```python
from build123d import *

# Parameters (mm, degrees)
F1_DEPTH    = 71.5
F0_R        = 0.8
F2_DEPTH    = 3
F3_T1_DEPTH = 18.8384580048
F3_T3_DEPTH = 18.8384580048
F3_T6_ANGLE = 198.9853445977
F3_T8_ANGLE = 161.0146554023
F6_W        = 6.8
F6_H        = 6.6
F7_DEPTH    = 10
F9_DEPTH    = 57.4


# Not quite as in the source:
# - a fillet or chamfer that OpenCascade refuses, or shapes differently, is made with other operations: its cross-section is extruded or revolved along the edge and cut away or added


with BuildPart() as f1:
    # F0 (on Top) → F1 (new body)
    with BuildSketch(Plane.XY):
        with BuildLine():
            ThreePointArc((10.5534817095, 15.4336250836), (0, 24.3689653978), (-10.5534817095, 15.4336250836))
            Line((-10.5534817095, 15.4336250836), (-13.6603478203, -3.1468722986))
            ThreePointArc((-13.6603478203, -3.1468722986), (0, -19.2810346022), (13.6603478203, -3.1468722986))
            Line((13.6603478203, -3.1468722986), (10.5534817095, 15.4336250836))
        make_face()
        with BuildLine():
            ThreePointArc((-12.1808877675, -3.3942544975), (-10.7458713669, 0.6557337165), (-8.0101498113, 3.9689653978))
            ThreePointArc((-8.0101498113, 3.9689653978), (-7.3298242511, 6.556361809), (-8.0101498113, 9.1437582202))
            ThreePointArc((-8.0101498113, 9.1437582202), (-9.0606365073, 12.0737017575), (-9.0740216568, 15.1862428847))
            ThreePointArc((-9.0740216568, 15.1862428847), (0, 22.8689653978), (9.0740216568, 15.1862428847))
            ThreePointArc((9.0740216568, 15.1862428847), (9.0606535532, 12.0737985759), (8.0102465186, 9.1439294077))
            ThreePointArc((8.0102465186, 9.1439294077), (8.0101981654, 9.1438438137), (8.0101498113, 9.1437582202))
            ThreePointArc((8.0101498113, 9.1437582202), (7.3298242511, 6.556361809), (8.0101498113, 3.9689653978))
            ThreePointArc((8.0101498113, 3.9689653978), (10.7458713669, 0.6557337165), (12.1808877675, -3.3942544975))
            ThreePointArc((12.1808877675, -3.3942544975), (0, -17.7810346022), (-12.1808877675, -3.3942544975))
        make_face(mode=Mode.SUBTRACT)
    extrude(amount=F1_DEPTH)

    # F0 (on Top) → F2 (join)
    with BuildSketch(Plane.XY):
        with BuildLine():
            ThreePointArc((10.5534817095, 15.4336250836), (0, 24.3689653978), (-10.5534817095, 15.4336250836))
            Line((-10.5534817095, 15.4336250836), (-13.6603478203, -3.1468722986))
            ThreePointArc((-13.6603478203, -3.1468722986), (0, -19.2810346022), (13.6603478203, -3.1468722986))
            Line((13.6603478203, -3.1468722986), (10.5534817095, 15.4336250836))
        make_face()
        with BuildLine():
            ThreePointArc((-12.1808877675, -3.3942544975), (-10.7458713669, 0.6557337165), (-8.0101498113, 3.9689653978))
            ThreePointArc((-8.0101498113, 3.9689653978), (-7.3298242511, 6.556361809), (-8.0101498113, 9.1437582202))
            ThreePointArc((-8.0101498113, 9.1437582202), (-9.0606365073, 12.0737017575), (-9.0740216568, 15.1862428847))
            ThreePointArc((-9.0740216568, 15.1862428847), (0, 22.8689653978), (9.0740216568, 15.1862428847))
            ThreePointArc((9.0740216568, 15.1862428847), (9.0606535532, 12.0737985759), (8.0102465186, 9.1439294077))
            ThreePointArc((8.0102465186, 9.1439294077), (8.0101981654, 9.1438438137), (8.0101498113, 9.1437582202))
            ThreePointArc((8.0101498113, 9.1437582202), (7.3298242511, 6.556361809), (8.0101498113, 3.9689653978))
            ThreePointArc((8.0101498113, 3.9689653978), (10.7458713669, 0.6557337165), (12.1808877675, -3.3942544975))
            ThreePointArc((12.1808877675, -3.3942544975), (0, -17.7810346022), (-12.1808877675, -3.3942544975))
        make_face(mode=Mode.SUBTRACT)
        with BuildLine():
            ThreePointArc((-9.0740216568, 15.1862428847), (-9.0606365073, 12.0737017575), (-8.0101498113, 9.1437582202))
            ThreePointArc((-8.0101498113, 9.1437582202), (0, 4.4689653978), (8.0101498113, 9.1437582202))
            ThreePointArc((8.0101498113, 9.1437582202), (8.0101981654, 9.1438438137), (8.0102465186, 9.1439294077))
            ThreePointArc((8.0102465186, 9.1439294077), (9.0606535532, 12.0737985759), (9.0740216568, 15.1862428847))
            ThreePointArc((9.0740216568, 15.1862428847), (0, 22.8689653978), (-9.0740216568, 15.1862428847))
        make_face()
        with BuildLine():
            ThreePointArc((-8.0101498113, 9.1437582202), (-7.3298242511, 6.556361809), (-8.0101498113, 3.9689653978))
            Line((-8.0101498113, 3.9689653978), (8.0101498113, 3.9689653978))
            ThreePointArc((8.0101498113, 3.9689653978), (7.3298242511, 6.556361809), (8.0101498113, 9.1437582202))
            ThreePointArc((8.0101498113, 9.1437582202), (0, 4.4689653978), (-8.0101498113, 9.1437582202))
        make_face()
        with BuildLine():
            Line((8.0101498113, 3.9689653978), (-8.0101498113, 3.9689653978))
            ThreePointArc((-8.0101498113, 3.9689653978), (-10.7458713669, 0.6557337165), (-12.1808877675, -3.3942544975))
            ThreePointArc((-12.1808877675, -3.3942544975), (0, -17.7810346022), (12.1808877675, -3.3942544975))
            ThreePointArc((12.1808877675, -3.3942544975), (10.7458713669, 0.6557337165), (8.0101498113, 3.9689653978))
        make_face()
        with Locations((-9, -5.4310346022)):
            Circle(F0_R, mode=Mode.SUBTRACT)
        with Locations((9, -5.4310346022)):
            Circle(F0_R, mode=Mode.SUBTRACT)
    extrude(amount=-F2_DEPTH)

    # F3: fillet of radius 6 on 1 edges, made by hand

    # F3_s2 → F3_t1 (cut)
    with BuildSketch(Plane(origin=(2.22343693, 13.2971819786, 0), x_dir=(0, 0, 1), z_dir=(-0.164921466, -0.9863067018, 0))):
        with BuildLine():
            ThreePointArc((-3, 6.9543058117), (-1.2426406871, 11.1969464988), (3, 12.9543058117))
            Line((3, 12.9543058117), (-3, 12.9543058117))
            Line((-3, 12.9543058117), (-3, 6.9543058117))
        make_face()
    extrude(amount=F3_T1_DEPTH, mode=Mode.SUBTRACT)

    # F3_s4 → F3_t3 (cut)
    with BuildSketch(Plane(origin=(0.8834291807, -5.2833154036, 0), x_dir=(0, 0, 1), z_dir=(-0.164921466, 0.9863067018, 0))):
        with BuildLine():
            ThreePointArc((3, 12.9543058117), (-1.2426406871, 11.1969464988), (-3, 6.9543058117))
            Line((-3, 6.9543058117), (-3, 12.9543058117))
            Line((-3, 12.9543058117), (3, 12.9543058117))
        make_face()
    extrude(amount=F3_T3_DEPTH, mode=Mode.SUBTRACT)

    # F3_s5 → F3_t6 (revolve, cut)
    with BuildSketch(Plane(origin=(-0.8834291807, -5.2833154036, 0), x_dir=(0, 0, 1), z_dir=(0.164921466, 0.9863067018, 0))):
        with BuildLine():
            ThreePointArc((-3, -6.9543058117), (-1.2426406871, -11.1969464988), (3, -12.9543058117))
            Line((3, -12.9543058117), (-3, -12.9543058117))
            Line((-3, -12.9543058117), (-3, -6.9543058117))
        make_face()
    revolve(axis=Axis((0, -5.4310346022, -3), (0, 0, 1)), revolution_arc=F3_T6_ANGLE, mode=Mode.SUBTRACT)

    # F3_s7 → F3_t8 (revolve, cut)
    with BuildSketch(Plane(origin=(-2.22343693, 13.2971819786, 0), x_dir=(0, 0, 1), z_dir=(0.164921466, -0.9863067018, 0))):
        with BuildLine():
            ThreePointArc((-3, -6.9543058117), (-1.2426406871, -11.1969464988), (3, -12.9543058117))
            Line((3, -12.9543058117), (-3, -12.9543058117))
            Line((-3, -12.9543058117), (-3, -6.9543058117))
        make_face()
    revolve(axis=Axis((0, 13.6689653978, -3), (0, 0, 1)), revolution_arc=F3_T8_ANGLE, mode=Mode.SUBTRACT)

    # F6 (on face) → F7 (cut)
    with BuildSketch(Plane(origin=(12.7769186395, 2.1364431051, 0), x_dir=(-0.164921466, 0.9863067018, 0), z_dir=(0.9863067018, 0.164921466, 0))):
        with Locations((4.8267343795, 16.4621602923)):
            Rectangle(F6_W, F6_H)
    extrude(amount=-F7_DEPTH, mode=Mode.SUBTRACT)

    # F8 (on face) → F9 (cut)
    with BuildSketch(Plane.XY.offset(71.5)):
        with BuildLine():
            Line((10.0688748062, 7.6421294361), (7.4430989219, 7.6421294361))
            ThreePointArc((7.4430989219, 7.6421294361), (7.3876854798, 5.7782940298), (7.9859788071, 4.0122254677))
            Line((7.9859788071, 4.0122254677), (10.6296725571, 4.4812676497))
            Line((10.6296725571, 4.4812676497), (10.0688748062, 7.6421294361))
        make_face()
    extrude(amount=-F9_DEPTH, mode=Mode.SUBTRACT)


solid = f1.part
```
Can you work these out from the model? Positions are in its coordinate system, mm. A direction names the side the tool comes from. Coordinates: 2 decimals unless noted, no trailing zeros. Answer as CSV lines item,"result".
Item 1: Please list where these lines run through material, in increasing order: line 1 along X through (y, z) = (-5, 12.5); line 2 along Z through (x, y) = (-3.75, 14.5); line 3 along X through (y, z) = (-7, 24).
Geometry results:
line 1,"x = -13.84 to -12.34, 12.34 to 13.84"
line 2,"z = -3 to 0"
line 3,"x = -13.76 to -12.25, 12.25 to 13.76"
Item 2: We'd pull the mould along X, two halves only. Please class faces 4 (the cylindrical face through (10.441, 5.731, -1.196)), 5 (the cylindrical face through (-8.26, -5.74, -1.47)), 6 (the cylindrical face through (0.21, 24.367, 37.73)): +X half, -X half, draft (parallel to the pull), parting line (faces both ways), or undercut.
Geometry results:
face 4,"+X half"
face 5,"undercut"
face 6,"parting line"
Item 3: I'm going to push flat-ended pins straight in: P1, Ø2, axis at x = -9, y = -5.43, coming from the +Z side; P2, Ø8, axis at x = 4.5, z = 32, coming from the -Y side; P3, Ø1.5, axis at x = 9.5, y = 8, coming from the -Z side. Where does each tip first touch, or does it pass through?
Geometry results:
P1,"stops at z = 0"
P2,"stops at y = -19.27"
P3,"stops at z = -2.2"
Item 4: On a 3-axis mill with a long thin cutter (end or side, diameter ignored), from which of +Z, -Z, +X, -X, +Y, -Y can I reach the whole of each face in a straight line? I mean faces 1 (the flat face through (9.889, 9.995, 16.416)), 2 (the flat face through (0, 3, -3)), 3 (the cylindrical face through (7.673, 8.425, 45.269)). Say none if no direction works.
Geometry results:
face 1,"+X"
face 2,"-Z, +X, -X, +Y, -Y"
face 3,"+Z"
